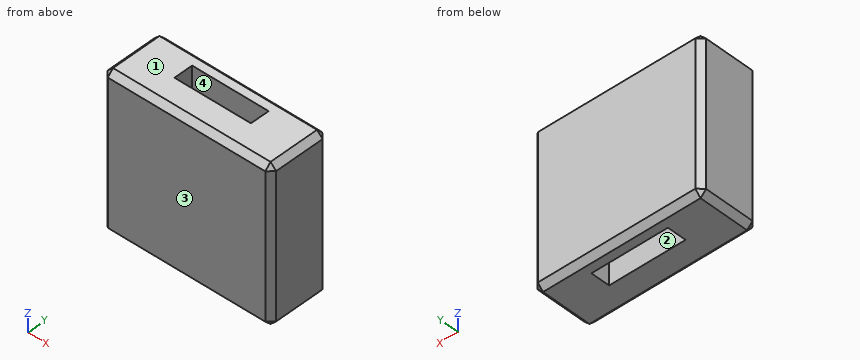
from build123d import *

# Parameters (mm, degrees)
F0_W     = 76.2
F0_H     = 27.6479
F0_W_2   = 34.544
F0_H_2   = 8.5852
F1_DEPTH = 69.85
F2_SIZE  = 2.54


with BuildPart() as f1:
    # F0 (on Top) → F1 (new body)
    with BuildSketch(Plane.XY):
        Rectangle(F0_W, F0_H)
        with Locations((0, 3.16865)):
            Rectangle(F0_W_2, F0_H_2, mode=Mode.SUBTRACT)
    extrude(amount=F1_DEPTH)

    # F2
    f2_edges = [f1.edges().sort_by_distance(p)[0] for p in [
        (38.1, -13.82395, 34.925),
        (-38.1, -13.82395, 34.925),
        (38.1, 13.82395, 34.925),
        (-38.1, 13.82395, 34.925),
        (0, 13.82395, 69.85),
        (0, -13.82395, 69.85),
        (0, -13.82395, 0),
        (0, 13.82395, 0),
        (-38.1, 0, 0),
        (38.1, 0, 0),
        (38.1, 0, 69.85),
        (-38.1, 0, 69.85),
    ]]
    chamfer(f2_edges, length=F2_SIZE)


solid = f1.part
Input: part model. Units: mm. Frame: model coordinates. Face numbers are marked on the shaded views. Give positions to 0.01 mm unless a question says otherwise; leave off trailing zeros. Write each loop counter-clockwise with the first axis right and the second up, starting at its lowest first coordinate (ties: lowest second). Pieces come first, ordered by that corner, then holes. Notation, with made-up numbers: (6.25, -35.5) -> (64.25, -35.5) arc R21 cw to (64.25, 2.5) -> close; hole circle Ø2 at (68.25, 85.5). An arc over 180 degrees is marked (long way). Use one line per item in the form item = value. Start each with the question number.
1) Section query B-B on y = 1. Return the cut outline in (x, z).
2) Ray query, probe 1 along Y at (x, z) = (-13.5, 45); probe 2 along X at (y, z) = (0.75, 26); probe 3 along X at (y, z) = (-11.75, 12). Return the intervals inside material, ascending. Write a range as from..to.
3) Section query A-A on x = -0.5. Return the cut outline in (y, z).
4) Draft query along Y for the marked faces 1, 2, 3 and 4. Return one class per face: pulls with the +Y half, pulls with the -Y half, needs draft (parallel to the pull), parting line crosses it, or undercut.
5) Section query C-C on z = 13. Return the cut outline in (x, y), then the cut area to 3 significant figures.
Outcome:
q1.outline = (-38.1, 2.54) -> (-35.56, 0) -> (-17.27, 0) -> (-17.27, 69.85) -> (-35.56, 69.85) -> (-38.1, 67.31) -> close; (17.27, 0) -> (35.56, 0) -> (38.1, 2.54) -> (38.1, 67.31) -> (35.56, 69.85) -> (17.27, 69.85) -> close
q2.probe_1 = -13.82..-1.12, 7.46..13.82
q2.probe_2 = -38.1..-17.27, 17.27..38.1
q2.probe_3 = -37.63..37.63
q3.outline = (-13.82, 2.54) -> (-11.28, 0) -> (-1.12, 0) -> (-1.12, 69.85) -> (-11.28, 69.85) -> (-13.82, 67.31) -> close; (7.46, 0) -> (11.28, 0) -> (13.82, 2.54) -> (13.82, 67.31) -> (11.28, 69.85) -> (7.46, 69.85) -> close
q4.face_1 = needs draft
q4.face_2 = undercut
q4.face_3 = pulls with the -Y half
q4.face_4 = undercut
q5.outline = (-38.1, -11.28) -> (-35.56, -13.82) -> (35.56, -13.82) -> (38.1, -11.28) -> (38.1, 11.28) -> (35.56, 13.82) -> (-35.56, 13.82) -> (-38.1, 11.28) -> close; hole (-17.27, -1.12) -> (17.27, -1.12) -> (17.27, 7.46) -> (-17.27, 7.46) -> close
q5.area = 1,800 mm^2
